The figure shows three views and two pictorial views of one solid part (mm, origin at its lowest corner). Answer the questions. A direction names the side the tool comes from. Give positions to 0.01 mm unless a question says otherwise; leave off trailing zeros. Write each loop counter-clockwise with the first axis right and the second up, starting at its lowest first coordinate (ties: lowest second). Pieces come first, ordered by that corner, then holes. Notation, with made-up numbers: M 24,-15 L 45,-15 A31 ccw 45,18 Z; hole C 71.25,-9.5 d11. An arc over 180 degrees is marked long. Return JSON: item names as keys, results as strings.
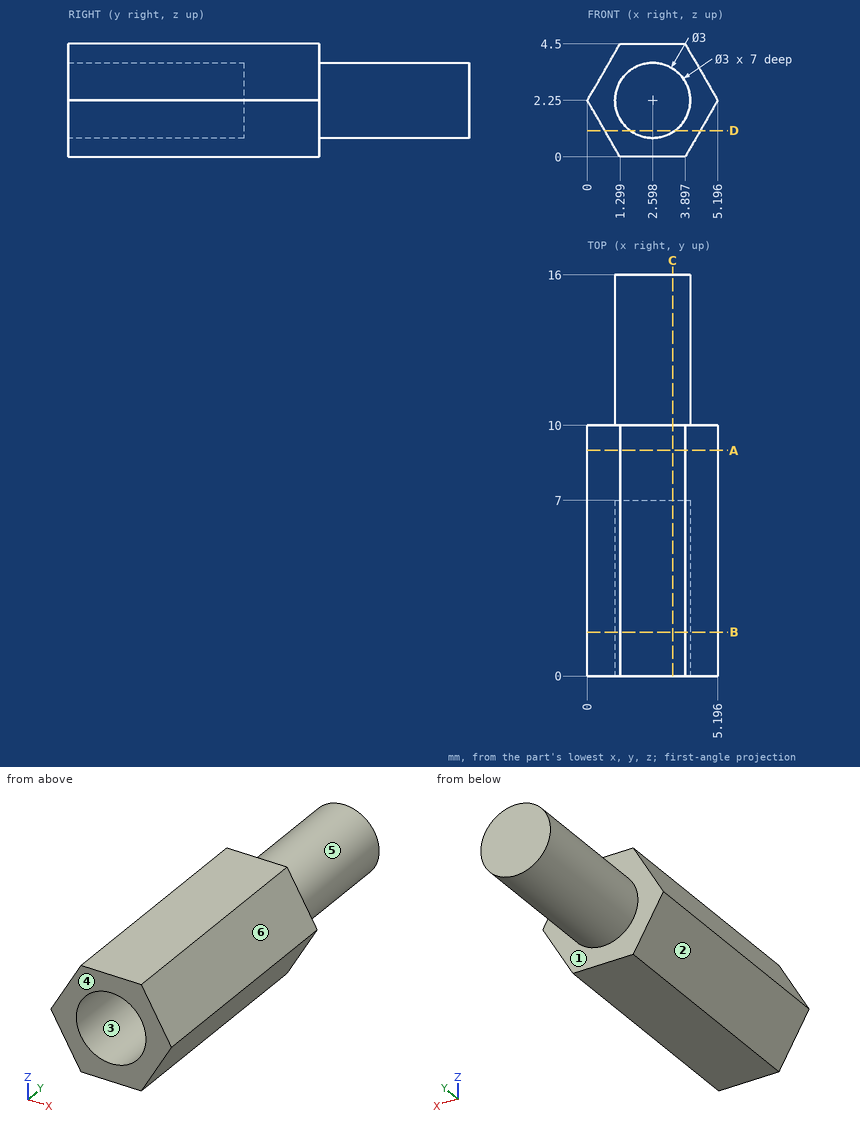
Item 1: A cutting plane is placed at C-C, the plane x = 3.4. Write down the section's boundary in (y, z).
Geometry results:
{"outline": "M 0,0 L 10,0 L 10,0.98 L 16,0.98 L 16,3.52 L 10,3.52 L 10,4.5 L 0,4.5 L 0,3.52 L 7,3.52 L 7,0.98 L 0,0.98 Z"}
Item 2: A cutting plane is placed at A-A, the plane y = 9. Write down the section's boundary in (x, z), plus the area to 3 significant figures.
Geometry results:
{"outline": "M 0,2.25 L 1.3,0 L 3.9,0 L 5.2,2.25 L 3.9,4.5 L 1.3,4.5 Z", "area": "17.5 mm2"}
Item 3: Determine the mould class of the marked faces 3, 4, 5 and 6 for opening direction X: +X half, -X half, draft (parallel to the pull), parting line (faces both ways), or undercut.
Geometry results:
{"face 3": "undercut", "face 4": "draft", "face 5": "parting line", "face 6": "+X half"}
Item 4: Given pin 1 Ø1.5 at (x, z) = (3, 2) entering from -Y; pin 2 Ø2 at (x, y) = (4, 8.5) entering from +Z, each flat-ended and moving along its own axis, determine where each tip first touches the part or whether it passes through.
Geometry results:
{"pin 1": "stops at y = 7", "pin 2": "stops at z = 4.5"}
Item 5: Find the intervals of material crossed by line 1 (Y direction, x = 1.05, z = 1.5); line 2 (Y direction, x = 1.7, z = 1.65); line 3 (Z direction, x = 1.8, y = 5), in increasing order.
Geometry results:
{"line 1": "y = 0 to 10", "line 2": "y = 7 to 16", "line 3": "z = 0 to 0.98, 3.52 to 4.5"}
Item 6: Which of the six approach directions +Z, -Z, +X, -X, +Y, -Y give full straight-line access (tool end or side, diameter ignored) to the marked faces 1 and 2?
Geometry results:
{"face 1": "+Y", "face 2": "-Z, -X, +Y, -Y"}
Item 7: A cutting plane is placed at D-D, the plane z = 1.05. Write down the section's boundary in (x, y), plus the area to 3 significant figures.
Geometry results:
{"outline": "M 0.69,0 L 1.7,0 L 1.7,7 L 3.5,7 L 3.5,0 L 4.5,0 L 4.5,10 L 3.5,10 L 3.5,16 L 1.7,16 L 1.7,10 L 0.69,10 Z", "area": "36.3 mm2"}
Item 8: A cutting plane is placed at B-B, the plane y = 1.75. Write down the section's boundary in (x, z).
Geometry results:
{"outline": "M 0,2.25 L 1.3,0 L 3.9,0 L 5.2,2.25 L 3.9,4.5 L 1.3,4.5 Z; hole C 2.6,2.25 d3"}
